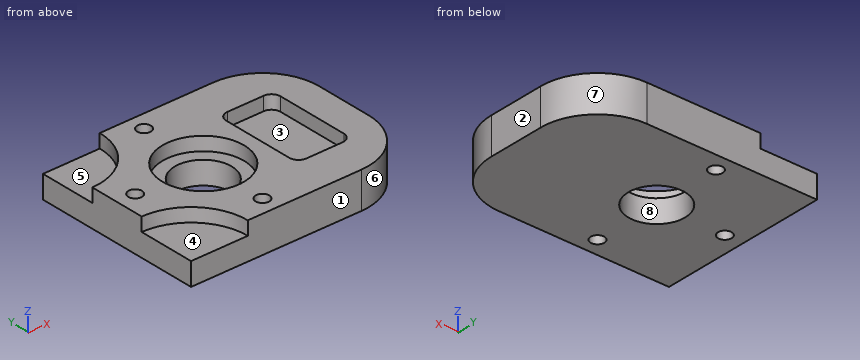
```python
from build123d import *

# Parameters (mm, degrees)
EXTRUDE1_DEPTH     = 16
SKETCH2_R          = 12.5
CUT_EXTRUDE1_DEPTH = 17
SKETCH3_R          = 18
CUT_EXTRUDE2_DEPTH = 6
SKETCH4_W          = 24
SKETCH4_H          = 40
CUT_EXTRUDE3_DEPTH = 6
FILLET1_R          = 4
HOLE1_D            = 6
SKETCH7_R          = 25
CUT_EXTRUDE4_DEPTH = 6


with BuildPart() as part:
    # Sketch1 → Extrude1 (new body)
    with BuildSketch(Plane.XY):
        with BuildLine():
            Line((0, 75), (75, 75))
            ThreePointArc((75, 75), (92.67766953, 67.67766953), (100, 50))
            Line((100, 50), (100, 25))
            ThreePointArc((100, 25), (92.67766953, 7.32233047), (75, 0))
            Line((75, 0), (0, 0))
            Line((0, 0), (0, 75))
        make_face()
    extrude(amount=EXTRUDE1_DEPTH)

    # Sketch2 → Cut-Extrude1 (cut, through all)
    with BuildSketch(Plane.XY.offset(16)):
        with Locations((38, 37.5)):
            Circle(SKETCH2_R)
    extrude(amount=-CUT_EXTRUDE1_DEPTH, mode=Mode.SUBTRACT)

    # Sketch3 → Cut-Extrude2 (cut)
    with BuildSketch(Plane.XY.offset(16)):
        with Locations((38, 37.5)):
            Circle(SKETCH3_R)
    extrude(amount=-CUT_EXTRUDE2_DEPTH, mode=Mode.SUBTRACT)

    # Sketch4 → Cut-Extrude3 (cut)
    with BuildSketch(Plane.XY.offset(16)):
        with Locations((74, 37.5)):
            Rectangle(SKETCH4_W, SKETCH4_H)
    extrude(amount=-CUT_EXTRUDE3_DEPTH, mode=Mode.SUBTRACT)

    # Fillet1
    fillet1_edges = [part.edges().sort_by_distance(p)[0] for p in [
        (62, 17.5, 13),
        (62, 57.5, 13),
        (86, 57.5, 13),
        (86, 17.5, 13),
    ]]
    fillet(fillet1_edges, radius=FILLET1_R)

    # Hole1 (through all)
    with Locations(Plane.XY.offset(16)):
        with Locations((38, 67.5), (8, 37.5), (38, 7.5)):
            Hole(HOLE1_D / 2)

    # Sketch7 → Cut-Extrude4 (cut)
    with BuildSketch(Plane.XY.offset(16)):
        with Locations((0, 75)):
            Circle(SKETCH7_R)
        Circle(SKETCH7_R)
    extrude(amount=-CUT_EXTRUDE4_DEPTH, mode=Mode.SUBTRACT)


solid = part.part
```
Part model, mm, in its own coordinate system. Face numbers are marked on the shaded views. A direction names the side the tool comes from. Coordinates: 2 decimals unless noted, no trailing zeros. Write each loop counter-clockwise with the first axis right and the second up, starting at its lowest first coordinate (ties: lowest second). Pieces come first, ordered by that corner, then holes.
Item 1: Slice it at C-C (x = 38). Write the cut outline in (y, z), and give its area (3 significant figures).
Item 2: Mould opens along Y. For the marked faces 6, 7 and 8 say: released by +Y, released by -Y, zero draft, split by the parting line, or undercut.
Item 3: Probe line 1 (Y direction, x = 8, z = 6.5); line 2 (Y direction, x = 38, z = 12.9); line 3 (Y direction, x = 38, z = 5). List the from-to ranges inside material, lowest first.
Item 4: Slice it at A-A (y = 37.5). Write the cut outline in (x, z), and give its area (3 significant figures).
Item 5: Slice it at D-D (z = 14.75). Write the cut outline in (x, y).
Item 6: Slice it at B-B (z = 4). Write the cut outline in (x, y), and give its area (3 significant figures).
Item 7: Pin check, flat tips, straight feed: pin 1 (9.5 mm diameter, centred on x = 38, y = 67.5, fed in from +Z); pin 2 (12 mm diameter, centred on x = 69.5, y = 41.5, fed in from +Z); pin 3 (1 mm diameter, centred on y = 22.5, z = 13, fed in from +X); pin 4 (3.5 mm diameter, centred on x = 8, y = 37.5, fed in from -Z). Stop position of each tip, or through.
Item 8: Which spindle directions (+Z, -Z, +X, -X, +Y, -Y) get a long thin tool onto all of the face, cutting with end or side? Do the marked faces 1, 2, 3, 4 and 5. Say none if no direction does.
Results found:
1. outline: (0, 0) - (4.5, 0) - (4.5, 16) - (0, 16) - close; (10.5, 0) - (25, 0) - (25, 10) - (19.5, 10) - (19.5, 16) - (10.5, 16) - close; (50, 0) - (64.5, 0) - (64.5, 16) - (55.5, 16) - (55.5, 10) - (50, 10) - close; (70.5, 0) - (75, 0) - (75, 16) - (70.5, 16) - close
1. area: 542 mm2
2. face 6: released by -Y
2. face 7: released by +Y
2. face 8: undercut
3. line 1: y = 0 to 34.5, 40.5 to 75
3. line 2: y = 0 to 4.5, 10.5 to 19.5, 55.5 to 64.5, 70.5 to 75
3. line 3: y = 0 to 4.5, 10.5 to 25, 50 to 64.5, 70.5 to 75
4. outline: (0, 0) - (5, 0) - (5, 16) - (0, 16) - close; (11, 0) - (25.5, 0) - (25.5, 10) - (20, 10) - (20, 16) - (11, 16) - close; (50.5, 0) - (100, 0) - (100, 16) - (86, 16) - (86, 10) - (62, 10) - (62, 16) - (56, 16) - (56, 10) - (50.5, 10) - close
4. area: 894 mm2
5. outline: (0, 25) arc R25 cw to (25, 0) - (75, 0) arc R25 ccw to (100, 25) - (100, 50) arc R25 ccw to (75, 75) - (25, 75) arc R25 cw to (0, 50) - close; hole circle Ø6 at (8, 37.5); hole circle Ø36 at (38, 37.5); hole circle Ø6 at (38, 7.5); hole circle Ø6 at (38, 67.5); hole (62, 21.5) arc R4 ccw to (66, 17.5) - (82, 17.5) arc R4 ccw to (86, 21.5) - (86, 53.5) arc R4 ccw to (82, 57.5) - (66, 57.5) arc R4 ccw to (62, 53.5) - close
6. outline: (0, 0) - (75, 0) arc R25 ccw to (100, 25) - (100, 50) arc R25 ccw to (75, 75) - (0, 75) - close; hole circle Ø6 at (8, 37.5); hole circle Ø25 at (38, 37.5); hole circle Ø6 at (38, 7.5); hole circle Ø6 at (38, 67.5)
6. area: 6,660 mm2
7. pin 1: stops at z = 16
7. pin 2: stops at z = 10
7. pin 3: stops at x = 99.92
7. pin 4: passes through
8. face 1: +Z, -Z, +X, -X, -Y
8. face 2: +Z, -Z, +X, +Y, -Y
8. face 3: +Z
8. face 4: +Z, -X, -Y
8. face 5: +Z, -X, +Y
